Autodesk Inventor part; units mm, degrees
ref_plane "YZ Plane" through (0, 0, 0) normal (1, 0, 0) x (0, 1, 0)
ref_plane "XZ Plane" through (0, 0, 0) normal (0, 1, 0) x (-1, 0, 0)
ref_plane "XY Plane" through (0, 0, 0) normal (0, 0, 1) x (1, 0, 0)
sketch "Sketch1" plane through (0, 0, 0) normal (0, 0, 1) x (1, 0, 0)
  line L0 (0, 8.2967) -> (5.8666, 5.8666)
  line L1 (5.8666, 5.8666) -> (8.2967, 0)
  line L2 (8.2967, 0) -> (5.8666, -5.8666)
  line L3 (5.8666, -5.8666) -> (0, -8.2967)
  line L4 (0, -8.2967) -> (-5.8666, -5.8666)
  line L5 (-5.8666, -5.8666) -> (-8.2967, 0)
  line L6 (-8.2967, 0) -> (-5.8666, 5.8666)
  line L7 (-5.8666, 5.8666) -> (0, 8.2967)
  line L8 (-81.026, 12.7) -> (12.7, 12.7)
  line L9 (12.7, 12.7) -> (12.7, -46.99)
  line L10 (12.7, -46.99) -> (-81.026, -46.99)
  line L11 (-81.026, -46.99) -> (-81.026, 12.7)
  point P0 (0, 0)
  point P1 (0, 0)
  dimension "d0" = 6.35
  dimension "d1" = 12.7
  dimension "d2" = 12.7
  dimension "d4" = 93.726
  dimension "d46" = 59.69
extrude "Extrusion1" add sketch "Sketch1" along normal blind 6.35
sketch "Sketch2" plane through (0, 0, 0) normal (0, 0, -1) x (-1, 0, 0)
  line L0 (81.026, -46.99) -> (-12.7, -46.99)
  line L1 (81.026, 12.7) -> (74.676, 12.7)
  line L2 (74.676, 12.7) -> (74.676, -46.99)
  line L3 (74.676, -46.99) -> (81.026, -46.99)
  line L4 (81.026, -46.99) -> (81.026, 12.7)
  point P0 (0, 0)
  dimension "d7" = 6.35
extrude "Extrusion2" add sketch "Sketch2" along normal blind 42.164
sketch "Sketch3" plane through (0, 0, -42.164) normal (0, 0, -1) x (-1, 0, 0)
  circle A0 centre (77.851, 7.62) radius 1.905
  circle A1 centre (77.851, -2.54) radius 1.905
  circle A2 centre (77.851, -12.7) radius 1.905
  circle A3 centre (77.851, -22.86) radius 1.905
  line L0 (81.026, -46.99) -> (81.026, 12.7)
  line L1 (81.026, 12.7) -> (74.676, 12.7)
  circle A4 centre (77.851, -33.02) radius 1.905
  circle A5 centre (77.851, -43.18) radius 1.905
  line L2 (74.676, -46.99) -> (81.026, -46.99)
  point P0 (0, 0)
  dimension "d10" = 3.81
  dimension "d11" = 3.175
  dimension "d12" = 5.08
  dimension "d13" = 3.81
  dimension "d14" = 3.175
  dimension "d15" = 10.16
  dimension "d16" = 3.81
  dimension "d17" = 10.16
  dimension "d18" = 3.175
  dimension "d19" = 3.81
  dimension "d20" = 3.175
  dimension "d21" = 10.16
  dimension "d26" = 3.81
  dimension "d27" = 3.175
  dimension "d28" = 3.81
  dimension "d29" = 10.16
  dimension "d30" = 3.175
  dimension "d31" = 3.81
  dimension "d43" = 10.16
extrude "Extrusion3" add sketch "Sketch3" along normal blind 3.81
sketch "Sketch4" plane through (0, 0, 0) normal (0, 0, -1) x (-1, 0, 0)
  line L0 (5.8666, 5.8666) -> (50.455, 5.8666)
  line L1 (74.676, 12.7) -> (-12.7, 12.7)
  line L2 (15.8582, 12.7) -> (28.5582, 12.7)
  line L3 (28.5582, 5.8666) -> (15.8582, 5.8666)
  line L4 (41.91, 12.7) -> (29.21, 12.7)
  line L5 (29.21, 12.7) -> (29.21, 5.8666)
  line L6 (29.21, 5.8666) -> (41.91, 5.8666)
  line L7 (41.91, 5.8666) -> (41.91, 12.7)
  line L8 (-12.7, 12.7) -> (-12.7, -46.99)
  line L9 (81.026, -46.99) -> (-12.7, -46.99)
  line L10 (35.56, -46.99) -> (41.91, -46.99)
  line L11 (41.91, -46.99) -> (41.91, -41.021)
  line L12 (41.91, -41.021) -> (35.56, -41.021)
  line L13 (35.56, -41.021) -> (35.56, -46.99)
  point P0 (0, 0)
  dimension "d35" = 12.7
  dimension "d36" = 41.91
  dimension "d49" = 6.35
  dimension "d50" = 5.969
  dimension "d51" = 48.26
extrude "Extrusion4" add sketch "Sketch4" along normal blind 6.35
sketch "Sketch5" plane through (-74.676, -46.99, 0) normal (1, 0, 0) x (0, 0, -1)
  line L0 (0, 52.8566) -> (28.7051, 52.8566)
  line L1 (0, 52.8566) -> (6.35, 52.8566)
  line L2 (0, 59.69) -> (42.164, 59.69)
  line L3 (19.05, 52.8566) -> (12.7, 52.8566)
  line L4 (12.7, 52.8566) -> (12.7, 59.69)
  line L5 (12.7, 59.69) -> (19.05, 59.69)
  line L6 (19.05, 59.69) -> (19.05, 52.8566)
  line L7 (-6.35, 0) -> (-6.35, 59.69)
  line L8 (0, 0) -> (42.164, 0)
  line L9 (-6.35, 0) -> (42.164, 0)
  line L10 (21.082, 0) -> (27.432, 0)
  line L11 (27.432, 0) -> (27.432, 5.969)
  line L12 (27.432, 5.969) -> (21.082, 5.969)
  line L13 (21.082, 5.969) -> (21.082, 0)
  point P0 (0, 46.99)
  dimension "d39" = 6.35
  dimension "d40" = 19.05
  dimension "d44" = 52.8566
  dimension "d45" = 6.8334
  dimension "d47" = 6.35
  dimension "d48" = 5.969
extrude "Extrusion5" add sketch "Sketch5" along normal blind 6.35
properties part number "polyoctpart"
Could you check a few things on this model? Use its own coordinates, in mm. A direction names the side the tool comes from. Round coordinates to 2 decimals unless told otherwise and drop trailing zeros. Order: outer loops, then holes, each group sorted by start corner. A loop starts at its lowest first (then second) coordinate and runs counter-clockwise, first axis right, second up. Notation, with made-up numbers: (-32.75, -24) -> (10.25, -24) arc R17 ccw to (10.25, -8) -> close; hole circle Ø2 at (1.25, 88.25). An arc over 180 degrees is marked (long way). One line per question, with ' | ' between items.
Q1. If we section it at B-B on y = -43.18: Write out the boundary of the cut face in (x, z).
Computed values:
outline: (-81.03, -42.16) -> (-79.76, -42.16) -> (-79.76, -45.97) -> (-75.95, -45.97) -> (-75.95, -42.16) -> (-74.68, -42.16) -> (-74.68, -27.43) -> (-68.33, -27.43) -> (-68.33, -21.08) -> (-74.68, -21.08) -> (-74.68, 0) -> (-41.91, 0) -> (-41.91, -6.35) -> (-35.56, -6.35) -> (-35.56, 0) -> (12.7, 0) -> (12.7, 6.35) -> (-81.03, 6.35) -> close
Q2. If we section it at C-C on y = 1: Write out the boundary of the cut face in (x, z).
Computed values:
outline: (-81.03, -42.16) -> (-74.68, -42.16) -> (-74.68, 0) -> (-7.88, 0) -> (-7.88, 6.35) -> (-81.03, 6.35) -> close; (7.88, 0) -> (12.7, 0) -> (12.7, 6.35) -> (7.88, 6.35) -> close
Q3. If I drill on line 1 (Z direction, x = -63, y = -35); line 2 (X direction, y = -35.5, z = -13); line 3 (Y direction, x = -5, z = 1), over which ranges is the centre line in solid material (lowest first)? Write a range as from..to.
Computed values:
line 1: 0..6.35 | line 2: -81.03..-74.68 | line 3: -46.99..-6.23, 6.23..12.7
Q4. I'm going to push flat-ended pins straight in: pin 1 (5 mm diameter, centred on x = -70.5, z = -15.5, fed in from -Y); pin 2 (7 mm diameter, centred on y = 7.5, z = -4, fed in from +X); pin 3 (10 mm diameter, centred on y = -1, z = -27, fed in from +X). Where does each tip first touch, or does it pass through?
Computed values:
pin 1: y = 5.87 | pin 2: x = -29.21 | pin 3: x = -74.68
Q5. If we section it at A-A on z = 1: Write out the boundary of the cut face in (x, y).
Computed values:
outline: (-81.03, -46.99) -> (12.7, -46.99) -> (12.7, 12.7) -> (-81.03, 12.7) -> close; hole (-8.3, 0) -> (-5.87, -5.87) -> (0, -8.3) -> (5.87, -5.87) -> (8.3, 0) -> (5.87, 5.87) -> (0, 8.3) -> (-5.87, 5.87) -> close
Q6. If we section it at D-D on x = -57: Write out the boundary of the cut face in (y, z), plus the area to 3 significant figures.
Computed values:
outline: (-46.99, 0) -> (12.7, 0) -> (12.7, 6.35) -> (-46.99, 6.35) -> close | area: 379 mm²
Q7. We'd pull the mould along X, two halves only. Please class faces 1 (the face through (-41.91, 9, -3)), 2 (the face through (-75.948, 7.536, -44.042)), 3 (the face through (-78, -33, -45.974)): released by +X, released by -X, zero draft, split by the parting line, or undercut.
Computed values:
face 1: undercut | face 2: split by the parting line | face 3: zero draft
Q8. Which directions (+Z, -Z, +X, -X, +Y, -Y) give clear straight access to the entire face, cutting with the end or side of a thin tool? Please do faces 4 (the face through (-78, -43, -45.974)), 5 (the face through (7.1, -2.89, 3.13)), 6 (the face through (-35, 9, -6.35)), 7 (the face through (-72, 5.867, -16)), 8 (the face through (-75.948, -2.624, -44.042)).
Computed values:
face 4: -Z, +X, -X, +Y, -Y | face 5: +Z, -Z | face 6: -Z, +X, +Y, -Y | face 7: -Z, +X, -Y | face 8: -Z
